Part model, mm, in its own coordinate system. Face numbers are marked on the shaded views. A direction names the side the tool comes from. Round coordinates to 2 decimals unless told otherwise and drop trailing zeros. Write each loop counter-clockwise with the first axis right and the second up, starting at its lowest first coordinate (ties: lowest second). Pieces come first, ordered by that corner, then holes. Notation, with made-up numbers: (-14, 16.5) -> (38, 16.5) arc R27 cw to (38, 38.5) -> close; hole circle Ø1 at (35, -19.75). An arc over 180 degrees is marked (long way). Use CSV: the item, a comma, the result in double quotes. Start each with the question number.
(1) Two-plate mould, pull along X, no slides. Class the marked faces 3, 4 and 5: released by +X, released by -X, zero draft, split by the parting line, or undercut.
(2) Drop a flat-ended pin along its axis: pin 1 (12 mm diameter, centred on x = 13, y = 25.5, fed in from +Z). Give the stop position or say it passes through.
(3) Which spindle directions (+Z, -Z, +X, -X, +Y, -Y) get a long thin tool onto all of the face, cutting with end or side? Do the marked faces 1 and 2. Say none if no direction does.
(4) Probe line 1 (Y direction, x = -12.5, z = -199); line 2 (X direction, y = 17, z = -253). List the from-to ranges inside material, lowest first. Write a range as [from, to].
(5) Saw through at C-C (x = 16). Give the cut face in (y, z), plus the area to 3 significant figures.
(6) Saw through at B-B (z = -160.5). Give the cut face in (x, y).
(7) Saw through at A-A (y = -6.5). Give the cut face in (x, z).
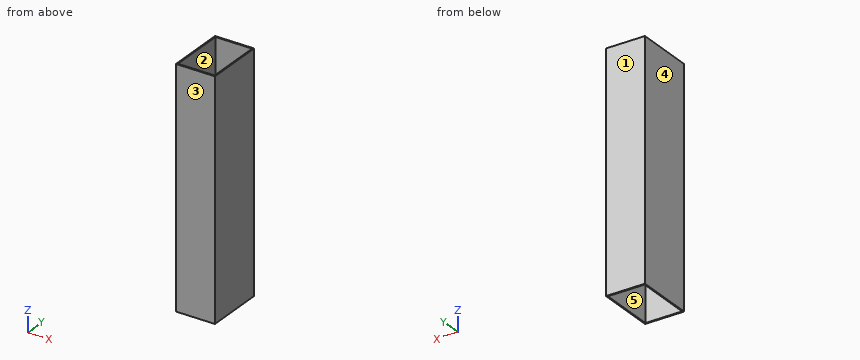
Autodesk Inventor part; units mm, degrees
ref_plane "YZ Plane" through (0, 0, 0) normal (1, 0, 0) x (0, 1, 0)
ref_plane "XZ Plane" through (0, 0, 0) normal (0, 1, 0) x (-1, 0, 0)
ref_plane "XY Plane" through (0, 0, 0) normal (0, 0, 1) x (1, 0, 0)
sketch "Sketch1" plane through (0, 0, 0) normal (0, 0, 1) x (1, 0, 0)
  line L0 (-25.4, -38.1) -> (25.4, -38.1)
  line L1 (25.4, -38.1) -> (25.4, 38.1)
  line L2 (25.4, 38.1) -> (-25.4, 38.1)
  line L3 (-25.4, 38.1) -> (-25.4, -38.1)
  line L4 (-25.4, -38.1) -> (25.4, 38.1) construction
  line L5 (25.4, -38.1) -> (-25.4, 38.1) construction
  line L6 (-23.8125, -36.5125) -> (23.8125, -36.5125)
  line L7 (23.8125, -36.5125) -> (23.8125, 36.5125)
  line L8 (23.8125, 36.5125) -> (-23.8125, 36.5125)
  line L9 (-23.8125, 36.5125) -> (-23.8125, -36.5125)
  line L10 (-23.8125, -36.5125) -> (23.8125, 36.5125) construction
  line L11 (23.8125, -36.5125) -> (-23.8125, 36.5125) construction
  point P0 (0, 0)
  dimension "d0" = 50.8
  dimension "d1" = 76.2
  dimension "d2" = 1.5875
  dimension "d3" = 1.5875
extrude "Extrusion1" add sketch "Sketch1" against normal blind 304.8
properties part number "2x3x1_16_rectangularTubing" material "Aluminum 6061"
Answers:
1,face 3,"zero draft"
1,face 4,"released by -X"
1,face 5,"undercut"
2,pin 1,"passes through"
3,face 1,"+Z, -Z, +X, -X, +Y"
3,face 2,"+Z, -Z"
4,line 1,"y = [-38.1, -36.51], [36.51, 38.1]"
4,line 2,"x = [-25.4, -23.81], [23.81, 25.4]"
5,outline,"(-38.1, -304.8) -> (-36.51, -304.8) -> (-36.51, 0) -> (-38.1, 0) -> close; (36.51, -304.8) -> (38.1, -304.8) -> (38.1, 0) -> (36.51, 0) -> close"
5,area,"968 mm²"
6,outline,"(-25.4, -38.1) -> (25.4, -38.1) -> (25.4, 38.1) -> (-25.4, 38.1) -> close; hole (-23.81, -36.51) -> (23.81, -36.51) -> (23.81, 36.51) -> (-23.81, 36.51) -> close"
7,outline,"(-25.4, -304.8) -> (-23.81, -304.8) -> (-23.81, 0) -> (-25.4, 0) -> close; (23.81, -304.8) -> (25.4, -304.8) -> (25.4, 0) -> (23.81, 0) -> close"
